Can you work these out from the model? Positions are in its coordinate system, mm. Face numbers are marked on the shaded views. Give positions to 0.01 mm unless a question says otherwise; leave off trailing zeros. Order: outer loops, then holes, each group sorted by start corner. A loop starts at its lowest first (then second) coordinate and runs counter-clockwise, first axis right, second up. Notation, with made-up numbers: (71.25, -12) -> (90.25, -12) arc R15 cw to (90.25, 14) -> close; hole circle Ø2 at (-15, -34.75). An arc over 180 degrees is marked (long way). Answer as CSV lines item,"result".
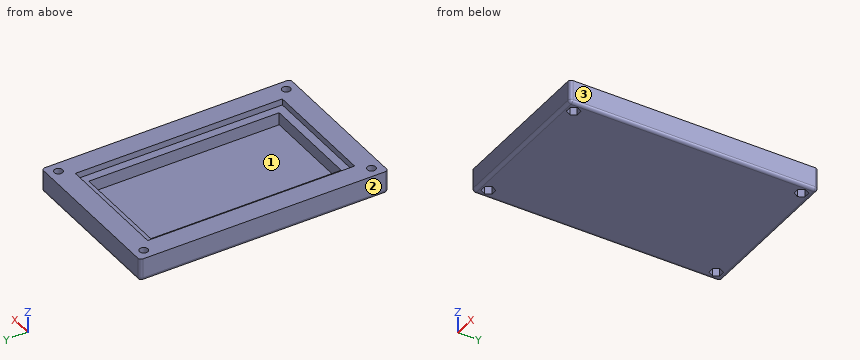
```python
from build123d import *

# Parameters (mm, degrees)
SKETCH001_W     = 37.94
SKETCH001_H     = 59.784
SKETCH001_R     = 1
PAD_DEPTH       = 5.5
SKETCH002_W     = 27.94
SKETCH002_H     = 49.784
POCKET_DEPTH    = 1.5
SKETCH_W        = 23.94
SKETCH_H        = 45.784
POCKET001_DEPTH = 3
POCKET002_DEPTH = 3
FILLET_R        = 0.75


with BuildPart() as part:
    # Sketch001 → Pad (new body)
    with BuildSketch(Plane.XY):
        Rectangle(SKETCH001_W, SKETCH001_H)
        with Locations((-16.47, 27.392)):
            Circle(SKETCH001_R, mode=Mode.SUBTRACT)
        with Locations((16.47, 27.392)):
            Circle(SKETCH001_R, mode=Mode.SUBTRACT)
        with Locations((-16.47, -27.392)):
            Circle(SKETCH001_R, mode=Mode.SUBTRACT)
        with Locations((16.47, -27.392)):
            Circle(SKETCH001_R, mode=Mode.SUBTRACT)
    extrude(amount=PAD_DEPTH)

    # Sketch002 (on Face10 of Pad) → Pocket (cut)
    with BuildSketch(Plane.XY.offset(5.5)):
        Rectangle(SKETCH002_W, SKETCH002_H)
    extrude(amount=-POCKET_DEPTH, mode=Mode.SUBTRACT)

    # Sketch (on Face15 of Pocket) → Pocket001 (cut)
    with BuildSketch(Plane.XY.offset(4)):
        Rectangle(SKETCH_W, SKETCH_H)
    extrude(amount=-POCKET001_DEPTH, mode=Mode.SUBTRACT)

    # Sketch003 (on Face4 of Pocket001) → Pocket002 (cut)
    with BuildSketch(Plane(origin=(0, 0, 0), x_dir=(1, 0, 0), z_dir=(0, 0, -1))):
        Polygon((-15.72, 26.092962), (-14.97, 27.392), (-15.72, 28.691038), (-17.22, 28.691038), (-17.97, 27.392), (-17.22, 26.092962), align=None)
        Polygon((17.22, 26.092962), (17.97, 27.392), (17.22, 28.691038), (15.72, 28.691038), (14.97, 27.392), (15.72, 26.092962), align=None)
        Polygon((-15.72, -28.691038), (-14.97, -27.392), (-15.72, -26.092962), (-17.22, -26.092962), (-17.97, -27.392), (-17.22, -28.691038), align=None)
        Polygon((17.22, -28.691038), (17.97, -27.392), (17.22, -26.092962), (15.72, -26.092962), (14.97, -27.392), (15.72, -28.691038), align=None)
    extrude(amount=-POCKET002_DEPTH, mode=Mode.SUBTRACT)

    # Fillet
    fillet_edges = [part.edges().sort_by_distance(p)[0] for p in [
        (0, -29.892, 0),
        (18.97, 0, 0),
        (18.97, 29.892, 2.75),
        (-18.97, -29.892, 2.75),
        (18.97, -29.892, 2.75),
        (0, 29.892, 0),
        (-18.97, 29.892, 2.75),
        (-18.97, 0, 0),
    ]]
    fillet(fillet_edges, radius=FILLET_R)


solid = part.part
```
Item 1: For pin 1 (22.5 mm diameter, centred on x = -1, y = 2.5, fed in from +Z), with a flat end and sliding along its axis, tell me the tip position at first contact or that it passes through.
Numbers:
pin 1,"stops at z = 4"
Item 2: Imagine slicing it at B-B, the plane x = -9. Please give me the cut outline in (y, z).
Numbers:
outline,"(-29.89, 0.75) arc R0.75 ccw to (-29.14, 0) -> (29.14, 0) arc R0.75 ccw to (29.89, 0.75) -> (29.89, 5.5) -> (24.89, 5.5) -> (24.89, 4) -> (22.89, 4) -> (22.89, 1) -> (-22.89, 1) -> (-22.89, 4) -> (-24.89, 4) -> (-24.89, 5.5) -> (-29.89, 5.5) -> close"
Item 3: Imagine slicing it at D-D, the plane z = 2.35. Give the number of separate pieces and of enclosed holes in the cut face, then the cut area to 3 significant figures.
Numbers:
separate pieces,"1"
enclosed holes,"5"
area,"1,150 mm²"
Item 4: Please list where these lines run through material, in increasing order: line 1 along Y through (x, z) = (-16.47, 4.8); line 2 along X through (y, z) = (6.5, 3.5); line 3 along Y through (x, z) = (-11, 4.1).
Numbers:
line 1,"y = -29.89 to -28.39, -26.39 to 26.39, 28.39 to 29.89"
line 2,"x = -18.97 to -11.97, 11.97 to 18.97"
line 3,"y = -29.89 to -24.89, 24.89 to 29.89"
Item 5: Imagine slicing it at C-C, the plane y = -11. Please give me the cut outline in (x, z), then the cut area to 3 significant figures.
Numbers:
outline,"(-18.97, 0.75) arc R0.75 ccw to (-18.22, 0) -> (18.22, 0) arc R0.75 ccw to (18.97, 0.75) -> (18.97, 5.5) -> (13.97, 5.5) -> (13.97, 4) -> (11.97, 4) -> (11.97, 1) -> (-11.97, 1) -> (-11.97, 4) -> (-13.97, 4) -> (-13.97, 5.5) -> (-18.97, 5.5) -> close"
area,"94.7 mm²"
Item 6: Imagine slicing it at A-A, the plane x = 16.47. Please give me the cut outline in (y, z).
Numbers:
outline,"(-29.89, 0.75) arc R0.75 ccw to (-29.14, 0) -> (-28.69, 0) -> (-28.69, 3) -> (-28.39, 3) -> (-28.39, 5.5) -> (-29.89, 5.5) -> close; (-26.39, 3) -> (-26.09, 3) -> (-26.09, 0) -> (26.09, 0) -> (26.09, 3) -> (26.39, 3) -> (26.39, 5.5) -> (-26.39, 5.5) -> close; (28.39, 3) -> (28.69, 3) -> (28.69, 0) -> (29.14, 0) arc R0.75 ccw to (29.89, 0.75) -> (29.89, 5.5) -> (28.39, 5.5) -> close"
Item 7: We'd pull the mould along X, two halves only. Please class the marked faces 1, 2 and 3: released by +X, released by -X, zero draft, split by the parting line, or undercut.
Numbers:
face 1,"undercut"
face 2,"released by -X"
face 3,"released by +X"
